```python
from build123d import *

# Parameters (mm, degrees)
SKETCH1_W                = 40
SKETCH1_H                = 40
BOSS_EXTRUDE1_DEPTH      = 40
SKETCH2_W                = 25
SKETCH2_H                = 20
CUT_EXTRUDE1_DEPTH       = 40
CHAMFER1_SIZE            = 15
CUT_EXTRUDE2_DEPTH       = 15
CHAMFER2_SIZE            = 4
SKETCH4_R                = 2.6
CUT_EXTRUDE3_DEPTH       = 17
BOSS_EXTRUDE2_DEPTH      = 8
BOSS_EXTRUDE2_DEPTH_BACK = 40
SKETCH5_W                = 40
SKETCH5_H                = 8.5
SKETCH5_H_2              = 5.5
SKETCH10_W               = 14
SKETCH10_H               = 10
CUT_EXTRUDE5_DEPTH       = 26
CHAMFER5_SIZE            = 8
SKETCH8_R                = 5.6
CUT_EXTRUDE4_DEPTH       = 34
BOSS_EXTRUDE3_DEPTH      = 20
FILLET3_R                = 4
FILLET4_R                = 2
SKETCH12_R               = 7
CUT_EXTRUDE6_DEPTH       = 1.5
CUT_EXTRUDE7_START       = -2.5
SKETCH13_R               = 7
CUT_EXTRUDE7_DEPTH       = 2.5
CHAMFER7_SIZE            = 25
FILLET6_R                = 8
CHAMFER8_SIZE            = 2
CHAMFER8_SIZE2           = 10
FILLET7_R                = 2
SKETCH14_W               = 40
SKETCH14_H               = 8.5
BOSS_EXTRUDE4_DEPTH      = 15
SKETCH15_R               = 4.3
CUT_EXTRUDE8_DEPTH       = 10
FILLET8_R                = 8
CHAMFER10_SIZE           = 0.5


with BuildPart() as part:
    # Sketch1 → Boss-Extrude1 (new body)
    with BuildSketch(Plane(origin=(0, 0, 0), x_dir=(1, 0, 0), z_dir=(0, 1, 0))):
        with Locations((20, 20)):
            Rectangle(SKETCH1_W, SKETCH1_H)
    extrude(amount=BOSS_EXTRUDE1_DEPTH)

    # Sketch2 → Cut-Extrude1 (cut)
    with BuildSketch(Plane(origin=(0, 40, 0), x_dir=(1, 0, 0), z_dir=(0, 1, 0))):
        with Locations((12.5, 30)):
            Rectangle(SKETCH2_W, SKETCH2_H)
    extrude(amount=-CUT_EXTRUDE1_DEPTH, mode=Mode.SUBTRACT)

    # Chamfer1
    chamfer1_edges = [part.edges().sort_by_distance(p)[0] for p in [
        (0, 20, 0),
    ]]
    chamfer(chamfer1_edges, length=CHAMFER1_SIZE)

    # Sketch3 → Cut-Extrude2 (cut)
    with BuildSketch(Plane.XY):
        Polygon((0, 10), (0, 15), (15, 15), (15, 5), (0, 5), align=None)
        Polygon((0, 30), (0, 25), (15, 25), (15, 35), (0, 35), align=None)
    extrude(amount=-CUT_EXTRUDE2_DEPTH, mode=Mode.SUBTRACT)

    # Chamfer2
    chamfer2_edges = [part.edges().sort_by_distance(p)[0] for p in [
        (15, 35, -7.5),
        (15, 25, -7.5),
        (15, 15, -7.5),
        (15, 5, -7.5),
    ]]
    chamfer(chamfer2_edges, length=CHAMFER2_SIZE)

    # Sketch4 → Cut-Extrude3 (cut)
    with BuildSketch(Plane.XY.offset(-15)):
        with Locations((8, 30)):
            Circle(SKETCH4_R)
        with Locations((8, 10)):
            Circle(SKETCH4_R)
    extrude(amount=-CUT_EXTRUDE3_DEPTH, mode=Mode.SUBTRACT)

    # Sketch5 → Boss-Extrude2 (add, two sides: drawn at the far end of the back side and taken through both)
    with BuildSketch(Plane(origin=(0, 0, -40), x_dir=(-1, 0, 0), z_dir=(0, 0, -1)).offset(-BOSS_EXTRUDE2_DEPTH_BACK)):
        with Locations((-60, 4.25)):
            Rectangle(SKETCH5_W, SKETCH5_H)
        with Locations((-60, 28.75)):
            Rectangle(SKETCH5_W, SKETCH5_H_2)
    extrude(amount=BOSS_EXTRUDE2_DEPTH + BOSS_EXTRUDE2_DEPTH_BACK)

    # Sketch10 → Cut-Extrude5 (cut)
    with BuildSketch(Plane(origin=(40, 0, 0), x_dir=(0, 0, -1), z_dir=(1, 0, 0))):
        with Locations((29, 20)):
            Rectangle(SKETCH10_W, SKETCH10_H)
    extrude(amount=-CUT_EXTRUDE5_DEPTH, mode=Mode.SUBTRACT)

    # Chamfer5
    chamfer5_edges = [part.edges().sort_by_distance(p)[0] for p in [
        (40, 28.75, -48),
    ]]
    chamfer(chamfer5_edges, length=CHAMFER5_SIZE - 0.0001)  # a hair under: the kernel refuses the full size

    # Sketch8 → Cut-Extrude4 (cut)
    with BuildSketch(Plane(origin=(0, 32, 0), x_dir=(1, 0, 0), z_dir=(0, 1, 0))):
        with Locations((65, 38)):
            Circle(SKETCH8_R)
    extrude(amount=-CUT_EXTRUDE4_DEPTH, mode=Mode.SUBTRACT)

    # Sketch9 → Boss-Extrude3 (add)
    with BuildSketch(Plane(origin=(40, 0, 0), x_dir=(0, 0, -1), z_dir=(1, 0, 0))):
        Polygon((0, 40), (0, 55), (4, 55), (20, 40), align=None)
        Polygon((0, 0), (0, -15), (4, -15), (20, 0), align=None)
    extrude(amount=-BOSS_EXTRUDE3_DEPTH)

    # Fillet3
    fillet3_edges = [part.edges().sort_by_distance(p)[0] for p in [
        (20, 55, -2),
        (40, 55, -2),
        (20, -15, -2),
        (40, -15, -2),
    ]]
    fillet(fillet3_edges, radius=FILLET3_R)

    # Fillet4
    fillet4_edges = [part.edges().sort_by_distance(p)[0] for p in [
        (32.5, 40, -40),
        (32.5, 0, -40),
    ]]
    fillet(fillet4_edges, radius=FILLET4_R)

    # Sketch12 → Cut-Extrude6 (cut)
    with BuildSketch(Plane(origin=(0, 31.5, 0), x_dir=(1, 0, 0), z_dir=(0, 1, 0))):
        with Locations(Location((65, 38, 0), (0, 0, 180))):
            Circle(SKETCH12_R)
    extrude(amount=-CUT_EXTRUDE6_DEPTH, mode=Mode.SUBTRACT)

    # Sketch13 → Cut-Extrude7 (cut)
    with BuildSketch(Plane.XZ.offset(CUT_EXTRUDE7_START)):
        with Locations(Location((65, -38, 0), (0, 0, 180))):
            Circle(SKETCH13_R)
    extrude(amount=CUT_EXTRUDE7_DEPTH, mode=Mode.SUBTRACT)

    # Chamfer7
    chamfer7_edges = [part.edges().sort_by_distance(p)[0] for p in [
        (80, 4.25, 0),
        (80, 28.75, 0),
    ]]
    chamfer(chamfer7_edges, length=CHAMFER7_SIZE)

    # Fillet6
    fillet6_edges = [part.edges().sort_by_distance(p)[0] for p in [
        (80, 28.75, -48),
        (47.9999, 28.75, -48),
        (55, 28.75, 0),
        (55, 4.25, 0),
        (80, 4.25, -25),
        (80, 28.75, -25),
    ]]
    fillet(fillet6_edges, radius=FILLET6_R)

    # Chamfer8
    chamfer8_edges = [part.edges().sort_by_distance(p)[0] for p in [
        (40, 20, -36),
    ]]
    chamfer8_side = [part.faces().sort_by_distance(p)[0] for p in [
        (40, 16.5625, -17.75),
    ]]
    chamfer(chamfer8_edges, length=CHAMFER8_SIZE, length2=CHAMFER8_SIZE2, reference=chamfer8_side[0])

    # Fillet7
    fillet7_edges = [part.edges().sort_by_distance(p)[0] for p in [
        (27.5, 15, -36),
        (32.5, 15, -22),
        (32.5, 25, -22),
        (27.5, 25, -36),
        (35, 25, -37),
        (35, 15, -37),
    ]]
    fillet(fillet7_edges, radius=FILLET7_R)

    # Sketch14 → Boss-Extrude4 (add)
    with BuildSketch(Plane(origin=(0, 0, -48), x_dir=(-1, 0, 0), z_dir=(0, 0, -1))):
        with Locations((-60, 4.25)):
            Rectangle(SKETCH14_W, SKETCH14_H)
    extrude(amount=BOSS_EXTRUDE4_DEPTH)

    # Sketch15 → Cut-Extrude8 (cut)
    with BuildSketch(Plane.XZ):
        with Locations(Location((65.260929409, -54.130501699, 0), (0, 0, 270))):
            Circle(SKETCH15_R)
        with Locations(Location((65.16900186, -21.868239994, 0), (0, 0, 270))):
            Circle(SKETCH15_R)
    extrude(amount=-CUT_EXTRUDE8_DEPTH, mode=Mode.SUBTRACT)

    # Fillet8
    fillet8_edges = [part.edges().sort_by_distance(p)[0] for p in [
        (80, 4.25, -63),
        (40, 4.25, -63),
    ]]
    fillet(fillet8_edges, radius=FILLET8_R)

    # Chamfer10
    chamfer10_edges = [part.edges().sort_by_distance(p)[0] for p in [
        (72, 31.5, -38),
        (72, 0, -38),
    ]]
    chamfer(chamfer10_edges, length=CHAMFER10_SIZE)


solid = part.part
```
Model file for the job. Use its own axes, mm. A direction names the side the tool comes from. Round coordinates to 2 decimals unless told otherwise and drop trailing zeros. Order: outer loops, then holes, each group sorted by start corner. A loop starts at its lowest first (then second) coordinate and runs counter-clockwise, first axis right, second up. Notation, with made-up numbers: (13, 4) -> (69, 4) arc R31 cw to (69, 29) -> close; hole circle Ø3 at (-21, -9). An arc over 180 degrees is marked (long way). Use one line per item in the form item = value.
Item 1: Flat gauge pins, fed straight in: pin 1 Ø1 at (x, y) = (17.5, 41.5) entering from +Z; pin 2 Ø1 at (y, z) = (30, -7.5) entering from -X; pin 3 Ø12 at (x, z) = (31, -33) entering from +Y; pin 4 Ø3 at (x, y) = (60.5, 29.5) entering from -Z. Where does each tip first touch, or does it go through?
Returned:
pin_1 = through
pin_2 = 15
pin_3 = 40
pin_4 = -48
Item 2: Cut at B-B, the plane y = 10. Write the cut outline in (x, z).
Returned:
outline = (0, -20) -> (5.4, -20) -> (5.4, -15) -> (0, -15) -> close; (10.6, -20) -> (25, -20) -> (25, -40) -> (40, -40) -> (40, 0) -> (15, 0) -> (15, -15) -> (10.6, -15) -> close
Item 3: Cut at A-A, the plane x = 8. Write the cut outline in (y, z), and give its area (3 significant figures).
Returned:
outline = (0, -20) -> (7.4, -20) -> (7.4, -15) -> (5, -15) -> (5, -7) -> (0, -7) -> close; (12.6, -20) -> (27.4, -20) -> (27.4, -15) -> (25, -15) -> (25, -7) -> (15, -7) -> (15, -15) -> (12.6, -15) -> close; (32.6, -20) -> (40, -20) -> (40, -7) -> (35, -7) -> (35, -15) -> (32.6, -15) -> close
area = 308 mm^2
Item 4: Drill centre lines: line 1 (X direction, y = 1.5, z = -38); line 2 (Y direction, x = 8, z = -16.2); line 3 (Y direction, x = 42, z = -38.5). Where is each one in solid material? Low to high.
Returned:
line_1 = 25 to 58, 72 to 80
line_2 = 0 to 7.4, 12.6 to 27.4, 32.6 to 40
line_3 = 0 to 8.5, 26 to 31.5
Item 5: Cut at C-C, the plane y = -5. Write the cut outline in (x, z).
Returned:
outline = (20, -14.67) -> (40, -14.67) -> (40, 0) -> (20, 0) -> close
Item 6: Tool access for faces 1 (the face through (12, 20, -20)), 2 (the face through (13, 33, -9)), 3 (the face through (60, 8.5, -31)), 4 (the face through (40, -4, -8)): list every direction of +Z, -Z, +X, -X, +Y, -Y with a clear straight run to the whole face (end or side of a thin tool).
Returned:
face_1 = -Z, -X, +Y, -Y
face_2 = +Z, -X
face_3 = +Z, -Z, +X
face_4 = +Z, -Z, +X, -Y
Item 7: Pull direction Y, two halves, no side cores. Call faces 5 (the face through (32, 40, -29)), 6 (the face through (40, 39, -16)), 7 (the face through (8, 5, -12)): released by +Y, released by -Y, zero draft, split by the parting line, or undercut.
Returned:
face_5 = released by +Y
face_6 = zero draft
face_7 = undercut
